Geometry check sheet. Reference: the model listing, model coordinates, mm. A direction names the side the tool comes from. Coordinates: 2 decimals unless noted, no trailing zeros. Order: outer loops, then holes, each group sorted by start corner. A loop starts at its lowest first (then second) coordinate and runs counter-clockwise, first axis right, second up. Notation, with made-up numbers: (39.25, 51) - (71.25, 51) arc R14 cw to (71.25, 60) - close; hole circle Ø6 at (26, -20.5). An arc over 180 degrees is marked (long way). Put each result on its own line as item: value.
from build123d import *

# Parameters (mm, degrees)
ESQUISSE1_W               = 200
ESQUISSE1_H               = 160
ESQUISSE1_R               = 5
ESQUISSE1_R_2             = 1.75
ESQUISSE1_W_2             = 10
ESQUISSE1_H_2             = 10
ESQUISSE1_H_3             = 30
BOSS_EXTRU_1_DEPTH        = 5
CONG_2_R                  = 1
ENL_V_MAT_EXTRU_1_DEPTH   = 129.16005618
ESQUISSE3_R               = 1.75
TROU_CUVE_DIRECTION_DEPTH = 129.16005618


with BuildPart() as part:
    # Esquisse1 → Boss.-Extru.1 (new body)
    with BuildSketch(Plane(origin=(0, 0, 0), x_dir=(0, 1, 0), z_dir=(0, 0, 1))):
        Rectangle(ESQUISSE1_W, ESQUISSE1_H)
        with Locations(Location((-75, 0, 0), (0, 0, 270))):
            Circle(ESQUISSE1_R, mode=Mode.SUBTRACT)
        with Locations(Location((-57.5, 35.5, 0), (0, 0, 270))):
            Circle(ESQUISSE1_R_2, mode=Mode.SUBTRACT)
        with Locations(Location((-57.5, -35.5, 0), (0, 0, 90))):
            Circle(ESQUISSE1_R_2, mode=Mode.SUBTRACT)
        with Locations(Location((65, 45, 0), (0, 0, 270))):
            Circle(ESQUISSE1_R_2, mode=Mode.SUBTRACT)
        with Locations(Location((65, -45, 0), (0, 0, 90))):
            Circle(ESQUISSE1_R_2, mode=Mode.SUBTRACT)
        with Locations(Location((-31, 37.5, 0), (0, 0, 270))):
            Circle(ESQUISSE1_R_2, mode=Mode.SUBTRACT)
        with Locations(Location((-31, 75, 0), (0, 0, 270))):
            Circle(ESQUISSE1_R_2, mode=Mode.SUBTRACT)
        with Locations(Location((6.5, 75, 0), (0, 0, 270))):
            Circle(ESQUISSE1_R_2, mode=Mode.SUBTRACT)
        with Locations(Location((6.5, 37.5, 0), (0, 0, 270))):
            Circle(ESQUISSE1_R_2, mode=Mode.SUBTRACT)
        with Locations(Location((-31, -46.541307377, 0), (0, 0, 270))):
            Circle(ESQUISSE1_R_2, mode=Mode.SUBTRACT)
        with Locations(Location((-31, -70.091307377, 0), (0, 0, 270))):
            Circle(ESQUISSE1_R_2, mode=Mode.SUBTRACT)
        with Locations(Location((15.5, -46.541307377, 0), (0, 0, 270))):
            Circle(ESQUISSE1_R_2, mode=Mode.SUBTRACT)
        with Locations(Location((15.5, -70.091307377, 0), (0, 0, 270))):
            Circle(ESQUISSE1_R_2, mode=Mode.SUBTRACT)
        with Locations(Location((-4.999283545, 0, 0), (0, 0, 270))):
            Circle(ESQUISSE1_R_2, mode=Mode.SUBTRACT)
        with Locations(Location((85, 33, 0), (0, 0, 270))):
            Circle(ESQUISSE1_R_2, mode=Mode.SUBTRACT)
        with Locations(Location((85.001189598, -32.999999989, 0), (0, 0, 270))):
            Circle(ESQUISSE1_R_2, mode=Mode.SUBTRACT)
        with Locations(Location((19, 33, 0), (0, 0, 270))):
            Circle(ESQUISSE1_R_2, mode=Mode.SUBTRACT)
        with Locations(Location((19.001189598, -32.999999989, 0), (0, 0, 270))):
            Circle(ESQUISSE1_R_2, mode=Mode.SUBTRACT)
        with Locations((-46, 35)):
            Rectangle(ESQUISSE1_W_2, ESQUISSE1_H_2, mode=Mode.SUBTRACT)
        with Locations((7, 0)):
            Rectangle(ESQUISSE1_W_2, ESQUISSE1_H_3, mode=Mode.SUBTRACT)
    extrude(amount=BOSS_EXTRU_1_DEPTH)

    # Congé2
    cong_2_edges = [part.edges().sort_by_distance(p)[0] for p in [
        (-40, -51, 2.5),
        (-30, -51, 2.5),
        (-30, -41, 2.5),
        (-40, -41, 2.5),
        (-15, 2, 2.5),
        (15, 2, 2.5),
        (15, 12, 2.5),
        (-15, 12, 2.5),
    ]]
    fillet(cong_2_edges, radius=CONG_2_R)

    # Esquisse2 → Enlèv. mat.-Extru.1 (cut, through all)
    with BuildSketch(Plane.XY.offset(5)):
        Polygon((-573.580399643, 598.167108478), (-698.698151963, -488.082468479), (684.299979338, -647.380682556), (762.904681953, 702.431902078), align=None)
        Polygon((-110, 40), (0, 160), (110, 40), (110, -40), (0, -160), (-110, -40), align=None, mode=Mode.SUBTRACT)
    extrude(amount=-ENL_V_MAT_EXTRU_1_DEPTH, mode=Mode.SUBTRACT)

    # Esquisse3 → Trou cuve direction (cut, through all)
    with BuildSketch(Plane(origin=(0, 0, 0), x_dir=(0, 1, 0), z_dir=(0, 0, 1))):
        with Locations(Location((-94.001515359, 0.004041019, 0), (0, 0, 270))):
            Circle(ESQUISSE3_R)
    extrude(amount=TROU_CUVE_DIRECTION_DEPTH, mode=Mode.SUBTRACT)


solid = part.part
Q1. Section check C-C on z = 3.05. State how many separate pieces and enclosed holes the cut face has, then the cut area to 3 significant figures.
Answer block:
separate pieces: 1
enclosed holes: 21
area: 30,000 mm^2
Q2. Draft check along Y on faces 3 (the flat face through (-1, -1, 0)), 4 (the flat face through (-67.68, 86.17, 2.54)), 5 (the flat face through (-35, -41, 2)). Enter one of: pulls with the +Y half, pulls with the -Y half, needs draft (parallel to the pull), parting line crosses it, or undercut.
Answer block:
face 3: needs draft
face 4: pulls with the +Y half
face 5: undercut
Q3. Access from +Z, -Z, +X, -X, +Y, -Y to the whole of each face (thin tool, end or side, straight path). Record for faces 1 (the flat face through (-80, -1, 2)), 2 (the flat face through (-15, 7, 2)).
Answer block:
face 1: +Z, -Z, -X, +Y, -Y
face 2: +Z, -Z
Q4. Section check A-A on y = -75. Record the boundary of the cut face in (x, z).
Answer block:
outline: (-77.92, 0) - (-5, 0) - (-5, 5) - (-77.92, 5) - close; (5, 0) - (77.92, 0) - (77.92, 5) - (5, 5) - close
Q5. Thickness scan on L1, parallel to Y at x = -33, z = 2.65; L2, parallel to Y at x = -35.5, z = 1.65; L3, parallel to Y at x = -37.5, z = 2.55. Record the ranges inside material, lowest first. Write a range as [from, to].
Answer block:
L1: y = [-100, -51], [-41, 17.25], [20.75, 83.25], [86.75, 100]
L2: y = [-100, -59.25], [-55.75, -51], [-41, 100]
L3: y = [-100, -51], [-41, -32.75], [-29.25, 4.75], [8.25, 100]
Q6. Section check B-B on x = -65. Record the boundary of the cut face in (y, z).
Answer block:
outline: (-89.09, 0) - (89.09, 0) - (89.09, 5) - (-89.09, 5) - close
